The model under review builds one solid part; all positions refer to its coordinate system, in mm. Face numbers are marked on the shaded views. A direction names the side the tool comes from. Round coordinates to 2 decimals unless told otherwise and drop trailing zeros. Write each loop counter-clockwise with the first axis right and the second up, starting at its lowest first coordinate (ties: lowest second). Pieces come first, ordered by that corner, then holes. Notation, with made-up numbers: (88.25, -11) -> (118.25, -11) arc R17 ccw to (118.25, 19) -> close; hole circle Ø7 at (18, 86). An arc over 180 degrees is marked (long way). Answer as a JSON object with one key per item and string values. Group by question number.
1) We need section C-C, the plane z = 1.4. Write out the cut boundary in (x, y), then the cut area to 3 significant figures.
2) We need section B-B, the plane y = -0.9. Write out the cut boundary in (x, z).
3) Mouldability with a two-part tool opening along X and no side actions: class the marked faces 3 and 4 as pulls with the +X half, pulls with the -X half, needs draft (parallel to the pull), parting line crosses it, or undercut.
4) Machinability: for the marked faces 1 and 2, which of the approach directions +Z, -Z, +X, -X, +Y, -Y give a long, thin tool a straight path to every point of the face, cutting with its end or side? Answer none if there is none.
5) We need section A-A, the plane x = 0. Write out the cut boundary in (y, z), then the cut area to 3 significant figures.
6) To check wall thickness, follow probe 1 along X at (y, z) = (-0.25, 0.4); probe 2 along Y at (x, z) = (0.05, -1.15); probe 3 along Y at (x, z) = (-0.65, -1.05). State the ranges of each line that lie inside material, in increasing order. Write a range as [from, to].
7) We need section D-D, the plane y = -0.15. Write out the cut boundary in (x, z), then the cut area to 3 significant figures.
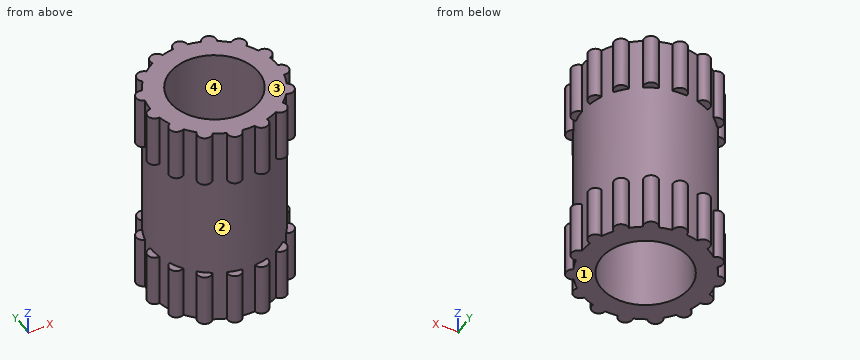
from build123d import *

# Parameters (mm, degrees)
SKETCH_R                     = 1.8
SKETCH_R_2                   = 1.25
PAD_DEPTH                    = 3
PAD_DEPTH_BACK               = 3
SKETCH001_R                  = 0.2
PAD001_DEPTH                 = 1.5
SKETCH001_POLARPATTERN_2_R   = 0.2
PAD001_POLARPATTERN_2_DEPTH  = 1.5
SKETCH001_POLARPATTERN_3_R   = 0.2
PAD001_POLARPATTERN_3_DEPTH  = 1.5
SKETCH001_POLARPATTERN_4_R   = 0.2
PAD001_POLARPATTERN_4_DEPTH  = 1.5
SKETCH001_POLARPATTERN_5_R   = 0.2
PAD001_POLARPATTERN_5_DEPTH  = 1.5
SKETCH001_POLARPATTERN_6_R   = 0.2
PAD001_POLARPATTERN_6_DEPTH  = 1.5
SKETCH001_POLARPATTERN_7_R   = 0.2
PAD001_POLARPATTERN_7_DEPTH  = 1.5
SKETCH001_POLARPATTERN_8_R   = 0.2
PAD001_POLARPATTERN_8_DEPTH  = 1.5
SKETCH001_POLARPATTERN_9_R   = 0.2
PAD001_POLARPATTERN_9_DEPTH  = 1.5
SKETCH001_POLARPATTERN_10_R  = 0.2
PAD001_POLARPATTERN_10_DEPTH = 1.5
SKETCH001_POLARPATTERN_11_R  = 0.2
PAD001_POLARPATTERN_11_DEPTH = 1.5
SKETCH001_POLARPATTERN_12_R  = 0.2
PAD001_POLARPATTERN_12_DEPTH = 1.5
SKETCH001_POLARPATTERN_13_R  = 0.2
PAD001_POLARPATTERN_13_DEPTH = 1.5
SKETCH001_POLARPATTERN_14_R  = 0.2
PAD001_POLARPATTERN_14_DEPTH = 1.5
SKETCH001_POLARPATTERN_15_R  = 0.2
PAD001_POLARPATTERN_15_DEPTH = 1.5


with BuildPart() as part:
    # Sketch → Pad (new body, two sides)
    with BuildSketch(Plane.XY) as pad_sk:
        Circle(SKETCH_R)
        Circle(SKETCH_R_2, mode=Mode.SUBTRACT)
    extrude(amount=PAD_DEPTH)
    extrude(pad_sk.sketch, amount=-PAD_DEPTH_BACK)

    # Sketch001 (on Face4 of Pad) → Pad001 (join)
    with BuildSketch(Plane.XY.offset(3)):
        with Locations((0, 1.8)):
            Circle(SKETCH001_R)
    pad001 = extrude(amount=-PAD001_DEPTH)

    # Sketch001 PolarPattern 2 → Pad001 PolarPattern 2 (add)
    with BuildSketch(Plane(origin=(0, 0, 3), x_dir=(0.913545, 0.406737, 0), z_dir=(0, 0, 1))):
        with Locations((0, 1.8)):
            Circle(SKETCH001_POLARPATTERN_2_R)
    pad001_polarpattern_2 = extrude(amount=-PAD001_POLARPATTERN_2_DEPTH)

    # Sketch001 PolarPattern 3 → Pad001 PolarPattern 3 (add)
    with BuildSketch(Plane(origin=(0, 0, 3), x_dir=(0.669131, 0.743145, 0), z_dir=(0, 0, 1))):
        with Locations((0, 1.8)):
            Circle(SKETCH001_POLARPATTERN_3_R)
    pad001_polarpattern_3 = extrude(amount=-PAD001_POLARPATTERN_3_DEPTH)

    # Sketch001 PolarPattern 4 → Pad001 PolarPattern 4 (add)
    with BuildSketch(Plane(origin=(0, 0, 3), x_dir=(0.309017, 0.951057, 0), z_dir=(0, 0, 1))):
        with Locations((0, 1.8)):
            Circle(SKETCH001_POLARPATTERN_4_R)
    pad001_polarpattern_4 = extrude(amount=-PAD001_POLARPATTERN_4_DEPTH)

    # Sketch001 PolarPattern 5 → Pad001 PolarPattern 5 (add)
    with BuildSketch(Plane(origin=(0, 0, 3), x_dir=(-0.104528, 0.994522, 0), z_dir=(0, 0, 1))):
        with Locations((0, 1.8)):
            Circle(SKETCH001_POLARPATTERN_5_R)
    pad001_polarpattern_5 = extrude(amount=-PAD001_POLARPATTERN_5_DEPTH)

    # Sketch001 PolarPattern 6 → Pad001 PolarPattern 6 (add)
    with BuildSketch(Plane(origin=(0, 0, 3), x_dir=(-0.5, 0.866025, 0), z_dir=(0, 0, 1))):
        with Locations((0, 1.8)):
            Circle(SKETCH001_POLARPATTERN_6_R)
    pad001_polarpattern_6 = extrude(amount=-PAD001_POLARPATTERN_6_DEPTH)

    # Sketch001 PolarPattern 7 → Pad001 PolarPattern 7 (add)
    with BuildSketch(Plane(origin=(0, 0, 3), x_dir=(-0.809017, 0.587785, 0), z_dir=(0, 0, 1))):
        with Locations((0, 1.8)):
            Circle(SKETCH001_POLARPATTERN_7_R)
    pad001_polarpattern_7 = extrude(amount=-PAD001_POLARPATTERN_7_DEPTH)

    # Sketch001 PolarPattern 8 → Pad001 PolarPattern 8 (add)
    with BuildSketch(Plane(origin=(0, 0, 3), x_dir=(-0.978148, 0.207912, 0), z_dir=(0, 0, 1))):
        with Locations((0, 1.8)):
            Circle(SKETCH001_POLARPATTERN_8_R)
    pad001_polarpattern_8 = extrude(amount=-PAD001_POLARPATTERN_8_DEPTH)

    # Sketch001 PolarPattern 9 → Pad001 PolarPattern 9 (add)
    with BuildSketch(Plane(origin=(0, 0, 3), x_dir=(-0.978148, -0.207912, 0), z_dir=(0, 0, 1))):
        with Locations((0, 1.8)):
            Circle(SKETCH001_POLARPATTERN_9_R)
    pad001_polarpattern_9 = extrude(amount=-PAD001_POLARPATTERN_9_DEPTH)

    # Sketch001 PolarPattern 10 → Pad001 PolarPattern 10 (add)
    with BuildSketch(Plane(origin=(0, 0, 3), x_dir=(-0.809017, -0.587785, 0), z_dir=(0, 0, 1))):
        with Locations((0, 1.8)):
            Circle(SKETCH001_POLARPATTERN_10_R)
    pad001_polarpattern_10 = extrude(amount=-PAD001_POLARPATTERN_10_DEPTH)

    # Sketch001 PolarPattern 11 → Pad001 PolarPattern 11 (add)
    with BuildSketch(Plane(origin=(0, 0, 3), x_dir=(-0.5, -0.866025, 0), z_dir=(0, 0, 1))):
        with Locations((0, 1.8)):
            Circle(SKETCH001_POLARPATTERN_11_R)
    pad001_polarpattern_11 = extrude(amount=-PAD001_POLARPATTERN_11_DEPTH)

    # Sketch001 PolarPattern 12 → Pad001 PolarPattern 12 (add)
    with BuildSketch(Plane(origin=(0, 0, 3), x_dir=(-0.104528, -0.994522, 0), z_dir=(0, 0, 1))):
        with Locations((0, 1.8)):
            Circle(SKETCH001_POLARPATTERN_12_R)
    pad001_polarpattern_12 = extrude(amount=-PAD001_POLARPATTERN_12_DEPTH)

    # Sketch001 PolarPattern 13 → Pad001 PolarPattern 13 (add)
    with BuildSketch(Plane(origin=(0, 0, 3), x_dir=(0.309017, -0.951057, 0), z_dir=(0, 0, 1))):
        with Locations((0, 1.8)):
            Circle(SKETCH001_POLARPATTERN_13_R)
    pad001_polarpattern_13 = extrude(amount=-PAD001_POLARPATTERN_13_DEPTH)

    # Sketch001 PolarPattern 14 → Pad001 PolarPattern 14 (add)
    with BuildSketch(Plane(origin=(0, 0, 3), x_dir=(0.669131, -0.743145, 0), z_dir=(0, 0, 1))):
        with Locations((0, 1.8)):
            Circle(SKETCH001_POLARPATTERN_14_R)
    pad001_polarpattern_14 = extrude(amount=-PAD001_POLARPATTERN_14_DEPTH)

    # Sketch001 PolarPattern 15 → Pad001 PolarPattern 15 (add)
    with BuildSketch(Plane(origin=(0, 0, 3), x_dir=(0.913545, -0.406737, 0), z_dir=(0, 0, 1))):
        with Locations((0, 1.8)):
            Circle(SKETCH001_POLARPATTERN_15_R)
    pad001_polarpattern_15 = extrude(amount=-PAD001_POLARPATTERN_15_DEPTH)

    # Mirrored: Pad001, Pad001 PolarPattern 2, Pad001 PolarPattern 3, Pad001 PolarPattern 4, Pad001 PolarPattern 5, Pad001 PolarPattern 6, Pad001 PolarPattern 7, Pad001 PolarPattern 8, Pad001 PolarPattern 9, Pad001 PolarPattern 10, Pad001 PolarPattern 11, Pad001 PolarPattern 12, Pad001 PolarPattern 13, Pad001 PolarPattern 14, Pad001 PolarPattern 15 across XY
    add(pad001.mirror(Plane.XY))
    add(pad001_polarpattern_2.mirror(Plane.XY))
    add(pad001_polarpattern_3.mirror(Plane.XY))
    add(pad001_polarpattern_4.mirror(Plane.XY))
    add(pad001_polarpattern_5.mirror(Plane.XY))
    add(pad001_polarpattern_6.mirror(Plane.XY))
    add(pad001_polarpattern_7.mirror(Plane.XY))
    add(pad001_polarpattern_8.mirror(Plane.XY))
    add(pad001_polarpattern_9.mirror(Plane.XY))
    add(pad001_polarpattern_10.mirror(Plane.XY))
    add(pad001_polarpattern_11.mirror(Plane.XY))
    add(pad001_polarpattern_12.mirror(Plane.XY))
    add(pad001_polarpattern_13.mirror(Plane.XY))
    add(pad001_polarpattern_14.mirror(Plane.XY))
    add(pad001_polarpattern_15.mirror(Plane.XY))


solid = part.part
Here are the results:
{
 "1": {"outline": "circle Ø3.6 at (0, 0); hole circle Ø2.5 at (0, 0)", "area": "5.27 mm^2"},
 "2": {"outline": "(-1.76, -3) -> (-0.87, -3) -> (-0.87, 3) -> (-1.76, 3) -> (-1.76, 1.5) -> (-1.56, 1.5) -> (-1.56, -1.5) -> (-1.76, -1.5) -> close; (0.87, -3) -> (1.76, -3) -> (1.76, -1.5) -> (1.56, -1.5) -> (1.56, 1.5) -> (1.76, 1.5) -> (1.76, 3) -> (0.87, 3) -> close"},
 "3": {"face 3": "needs draft", "face 4": "undercut"},
 "4": {"face 1": "-Z, +X, -X, +Y, -Y", "face 2": "none"},
 "5": {"outline": "(-1.8, -3) -> (-1.25, -3) -> (-1.25, 3) -> (-1.8, 3) -> close; (1.25, -3) -> (2, -3) -> (2, -1.5) -> (1.8, -1.5) -> (1.8, 1.5) -> (2, 1.5) -> (2, 3) -> (1.25, 3) -> close", "area": "7.20 mm^2"},
 "6": {"probe 1": "x = [-1.78, -1.22], [1.22, 1.78]", "probe 2": "y = [-1.8, -1.25], [1.25, 1.8]", "probe 3": "y = [-1.68, -1.07], [1.07, 1.68]"},
 "7": {"outline": "(-1.99, -3) -> (-1.24, -3) -> (-1.24, 3) -> (-1.99, 3) -> (-1.99, 1.5) -> (-1.79, 1.5) -> (-1.79, -1.5) -> (-1.99, -1.5) -> close; (1.24, -3) -> (1.99, -3) -> (1.99, -1.5) -> (1.79, -1.5) -> (1.79, 1.5) -> (1.99, 1.5) -> (1.99, 3) -> (1.24, 3) -> close", "area": "7.79 mm^2"}
}
